```python
from build123d import *

# Parameters (mm, degrees)
SKETCH_R      = 11
SKETCH_R_2    = 4.75
PAD_DEPTH     = 0.9
SKETCH001_R   = 6.5
SKETCH001_R_2 = 4.75
PAD001_DEPTH  = 1.8
CHAMFER_SIZE  = 0.3


with BuildPart() as part:
    # Sketch → Pad (new body)
    with BuildSketch(Plane.XY):
        Circle(SKETCH_R)
        Circle(SKETCH_R_2, mode=Mode.SUBTRACT)
    extrude(amount=PAD_DEPTH)

    # Sketch001 (on Face4 of Pad) → Pad001 (join)
    with BuildSketch(Plane.XY.offset(0.9)):
        Circle(SKETCH001_R)
        Circle(SKETCH001_R_2, mode=Mode.SUBTRACT)
    extrude(amount=PAD001_DEPTH)

    # Chamfer
    chamfer_edges = [part.edges().sort_by_distance(p)[0] for p in [
        (-6.5, 0, 2.7),
    ]]
    chamfer(chamfer_edges, length=CHAMFER_SIZE)


solid = part.part
```
The model under review builds one solid part; all positions refer to its coordinate system, in mm. A direction names the side the tool comes from. Round coordinates to 2 decimals unless told otherwise and drop trailing zeros. Order: outer loops, then holes, each group sorted by start corner. A loop starts at its lowest first (then second) coordinate and runs counter-clockwise, first axis right, second up. Notation, with made-up numbers: M -10,53.5 L 3,53.5 A6 cw 3,58.5 Z; hole C 67,78.5 d9. An arc over 180 degrees is marked long. Use a Markdown table: item, result.
1) Tool access review of faces 1 (the face through (-1, -5, 2.7)), 2 (the face through (-5.158, -3.955, 1.64)): name each direction out of +Z, -Z, +X, -X, +Y, -Y from which nothing blocks a thin tool from reaching the whole face with its end or side.
Report:
| item | result |
|---|---|
| face 1 | +Z, +X, -X, +Y, -Y |
| face 2 | +Z |
2) Consider section D-D (y = -9). Write out the cut boundary in (x, z).
Report:
| item | result |
|---|---|
| outline | M -6.32,0 L 6.32,0 L 6.32,0.9 L -6.32,0.9 Z |
3) Insertion check: pin 1 (1.5 mm diameter, centred on y = -4.5, z = 1, fed in from +X); pin 2 (1 mm diameter, centred on x = -3.5, z = 2, fed in from -Y). Each pin has a flat end and moves straight along its axis. Give the tip position at first contact, or say it passes through.
Report:
| item | result |
|---|---|
| pin 1 | x = 10.34 |
| pin 2 | y = -5.77 |
4) Consider section C-C (z = 1.2). Write out the cut boundary in (x, y).
Report:
| item | result |
|---|---|
| outline | C 0,0 d13; hole C 0,0 d9.5 |
5) Wall thickness on line 1 along Y through (x, z) = (0, 1.35); line 2 along Y through (x, z) = (2.25, 0.2); line 3 along Z through (x, y) = (-1.75, 7.5): over which ranges is each line inside the solid? List them lowest first. Write a range as [from, to].
Report:
| item | result |
|---|---|
| line 1 | [-6.5, -4.75], [4.75, 6.5] |
| line 2 | [-10.77, -4.18], [4.18, 10.77] |
| line 3 | [0, 0.9] |
6) Draft analysis for pull direction Y (two halves, no side actions). For faces 3 (the face through (2.192, -4.214, 1.331)), 4 (the face through (-2.38, -10.74, 0.44)), 5 (the face through (2, -5, 0)), state which applies: released by +Y, released by -Y, zero draft, split by the parting line, or undercut.
Report:
| item | result |
|---|---|
| face 3 | undercut |
| face 4 | split by the parting line |
| face 5 | zero draft |
7) Consider section A-A (x = 0). Write out the cut boundary in (y, z).
Report:
| item | result |
|---|---|
| outline | M -11,0 L -4.75,0 L -4.75,2.7 L -6.2,2.7 L -6.5,2.4 L -6.5,0.9 L -11,0.9 Z; M 4.75,0 L 11,0 L 11,0.9 L 6.5,0.9 L 6.5,2.4 L 6.2,2.7 L 4.75,2.7 Z |
